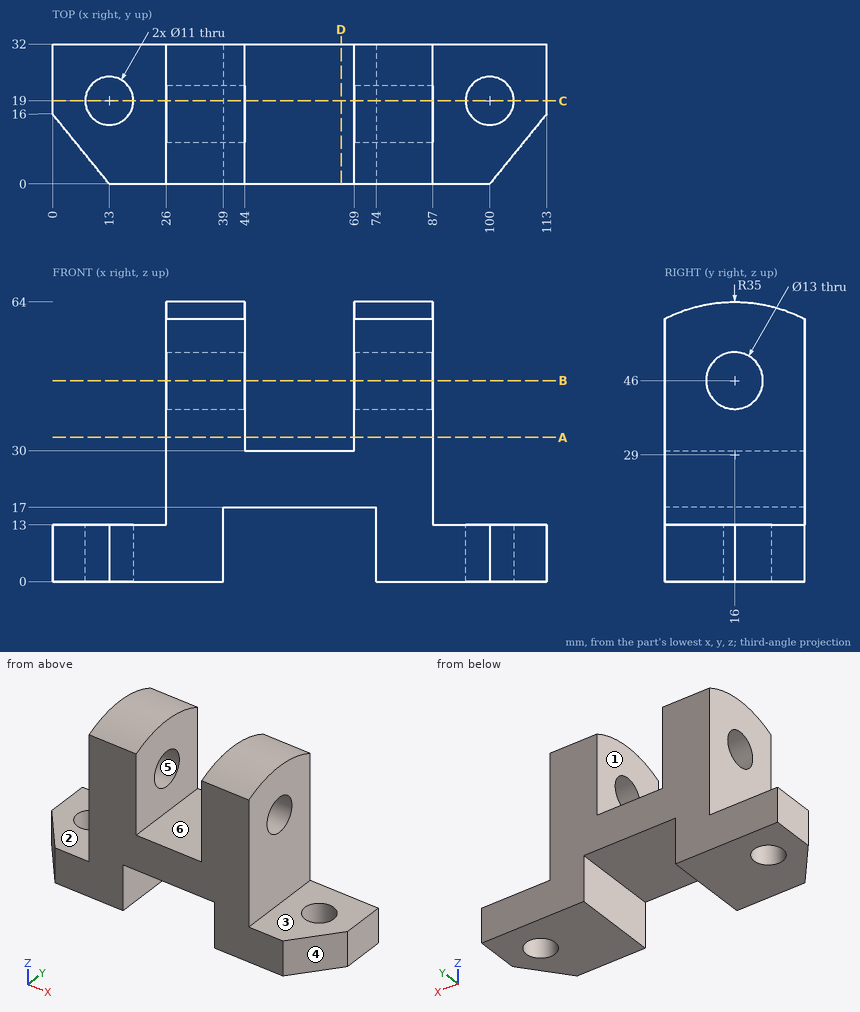
Input: dimensioned drawing with shaded views. Units: mm. Origin: part minimum x, y, z. A direction names the side the tool comes from. Round coordinates to 2 decimals unless told otherwise and drop trailing zeros. Loops run counter-clockwise (first coordinate to the right, second up) from the corner with the lowest first, then second, coordinate; pieces in that order, holes last. Notation, with made-up numbers: (11, 19) -> (39, 19) arc R23 cw to (39, 43) -> close; hole circle Ø7 at (45.5, -26). An arc over 180 degrees is marked (long way). Answer as a JSON object with one key per item and string values. Group by question number.
Q1. Access query for the marked faces 1, 2 and 3. Directions: +Z, -Z, +X, -X, +Y, -Y. A direction counts if a zero-diameter tool reaches every point of the face in a straight line with its end or side. Return the directions, or none.
Q2. Contact query for flat-ended pins moving along their axis: P1, Ø9.5, axis at x = 55.5, y = 22, coming from the -Z side; P2, Ø4, axis at y = 20.5, z = 21.5, coming from the -X side; P3, Ø12.5, axis at x = 55, y = 14, coming from the +Z side; P4, Ø18.5, axis at y = 12.5, z = 10.5, coming from the -X side. Output: stop coordinate, or through.
Q3. Section query A-A (z = 33). Output: boundary loops of the cut face in (x, y), plus the area to 3 significant figures.
Q4. Ray query, line 1 (Y direction, x = 13, z = 6.5); line 2 (X direction, y = 28.5, z = 7.5); line 3 (X direction, y = 7, z = 47). Return the intervals inside material, ascending. Write a range as from..to.
Q5. Section query B-B (z = 46). Output: boundary loops of the cut face in (x, y).
Q6. Mould query, pull axis Y, two halves, no side actions, for the marked faces 4, 5 and 6. Classes: pulls with the +Y half, pulls with the -Y half, needs draft (parallel to the pull), parting line crosses it, or undercut.
Q7. Section query D-D (x = 66). Output: boundary loops of the cut face in (y, z), plus the area to 3 significant figures.
Q8. Section query C-C (y = 19). State how many separate pieces and enclosed holes the cut face has, plus the area to 3 significant figures.
Completed:
{
 "1": {"face 1": "+Z, +Y, -Y", "face 2": "+Z, -X, +Y, -Y", "face 3": "+Z, +X, +Y, -Y"},
 "2": {"P1": "z = 17", "P2": "x = 26", "P3": "z = 30", "P4": "x = 0"},
 "3": {"outline": "(26, 0) -> (44, 0) -> (44, 32) -> (26, 32) -> close; (69, 0) -> (87, 0) -> (87, 32) -> (69, 32) -> close", "area": "1,150 mm²"},
 "4": {"line 1": "0..13.5, 24.5..32", "line 2": "0..39, 74..113", "line 3": "26..44, 69..87"},
 "5": {"outline": "(26, 0) -> (44, 0) -> (44, 9.5) -> (26, 9.5) -> close; (26, 22.5) -> (44, 22.5) -> (44, 32) -> (26, 32) -> close; (69, 0) -> (87, 0) -> (87, 9.5) -> (69, 9.5) -> close; (69, 22.5) -> (87, 22.5) -> (87, 32) -> (69, 32) -> close"},
 "6": {"face 4": "pulls with the -Y half", "face 5": "undercut", "face 6": "needs draft"},
 "7": {"outline": "(0, 17) -> (32, 17) -> (32, 30) -> (0, 30) -> close", "area": "416 mm²"},
 "8": {"separate pieces": "5", "enclosed holes": "0", "area": "2,430 mm²"}
}
